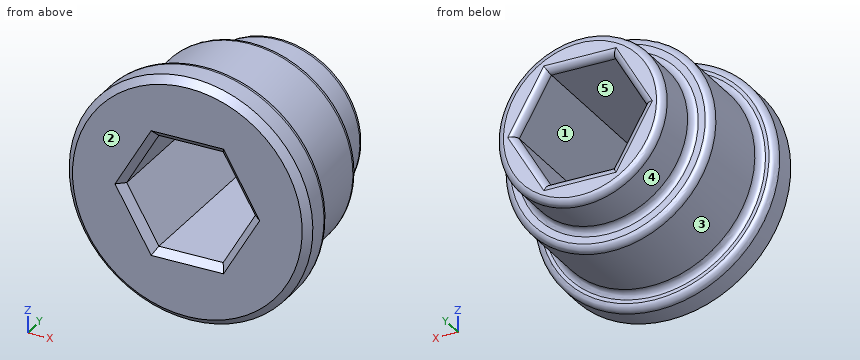
from build123d import *

# Parameters (mm, degrees)
SKETCH1_R           = 9.525
BOSS_EXTRUDE1_DEPTH = 7.9375
SKETCH2_R           = 7.62
BOSS_EXTRUDE2_DEPTH = 4.7625
SKETCH3_R           = 11.1125
BOSS_EXTRUDE3_DEPTH = 3.175
FILLET1_R           = 0.635
FILLET3_R           = 0.635
FILLET4_R           = 0.635
CHAMFER1_SIZE       = 0.635


with BuildPart() as part:
    # Sketch1 → Boss-Extrude1 (new body)
    with BuildSketch(Plane(origin=(0, 0, 0), x_dir=(1, 0, 0), z_dir=(0, 1, 0))):
        with Locations(Location((0, 0, 0), (0, 0, 270))):
            Circle(SKETCH1_R)
        Polygon((5.865878735, 0), (2.932939367, 5.08), (-2.932939367, 5.08), (-5.865878735, 0), (-2.932939367, -5.08), (2.932939367, -5.08), align=None, mode=Mode.SUBTRACT)
    extrude(amount=BOSS_EXTRUDE1_DEPTH)

    # Sketch2 → Boss-Extrude2 (add)
    with BuildSketch(Plane(origin=(0, 7.9375, 0), x_dir=(1, 0, 0), z_dir=(0, 1, 0))):
        with Locations(Location((0, 0, 0), (0, 0, 90))):
            Circle(SKETCH2_R)
        Polygon((-2.932939367, 5.08), (-5.865878735, 0), (-2.932939367, -5.08), (2.932939367, -5.08), (5.865878735, 0), (2.932939367, 5.08), align=None, mode=Mode.SUBTRACT)
    extrude(amount=BOSS_EXTRUDE2_DEPTH)

    # Sketch3 → Boss-Extrude3 (add)
    with BuildSketch(Plane.XZ):
        with Locations(Location((0, 0, 0), (0, 0, 270))):
            Circle(SKETCH3_R)
        Polygon((-2.932939367, 5.08), (2.932939367, 5.08), (5.865878735, 0), (2.932939367, -5.08), (-2.932939367, -5.08), (-5.865878735, 0), align=None, mode=Mode.SUBTRACT)
    extrude(amount=BOSS_EXTRUDE3_DEPTH)

    # Fillet1
    fillet1_edges = [part.edges().sort_by_distance(p)[0] for p in [
        (0, 0, -9.525),
        (0, 0, 11.1125),
    ]]
    fillet(fillet1_edges, radius=FILLET1_R)

    # Fillet3
    fillet3_edges = [part.edges().sort_by_distance(p)[0] for p in [
        (0, 12.7, -5.08),
        (-4.399409051, 12.7, -2.54),
        (-4.399409051, 12.7, 2.54),
        (0, 12.7, 5.08),
        (4.399409051, 12.7, 2.54),
        (4.399409051, 12.7, -2.54),
    ]]
    fillet(fillet3_edges, radius=FILLET3_R)

    # Fillet4
    fillet4_edges = [part.edges().sort_by_distance(p)[0] for p in [
        (0, 12.7, 7.62),
        (0, 7.9375, 7.62),
        (0, 7.9375, -9.525),
    ]]
    fillet(fillet4_edges, radius=FILLET4_R)

    # Chamfer1
    chamfer1_edges = [part.edges().sort_by_distance(p)[0] for p in [
        (0, -3.175, 11.1125),
        (-4.399409051, -3.175, 2.54),
        (-4.399409051, -3.175, -2.54),
        (0, -3.175, -5.08),
        (4.399409051, -3.175, -2.54),
        (4.399409051, -3.175, 2.54),
        (0, -3.175, 5.08),
    ]]
    chamfer(chamfer1_edges, length=CHAMFER1_SIZE)


solid = part.part
Geometry check sheet. Reference: the model listing, model coordinates, mm. Face numbers are marked on the shaded views. A direction names the side the tool comes from. Give positions to 0.01 mm unless a question says otherwise; leave off trailing zeros. Write each loop counter-clockwise with the first axis right and the second up, starting at its lowest first coordinate (ties: lowest second). Pieces come first, ordered by that corner, then holes. Notation, with made-up numbers: (-28.5, 46) - (-6.5, 46) arc R9 ccw to (-6.5, 58) - close; hole circle Ø8 at (61.25, 62). An arc over 180 degrees is marked (long way). Put each result on its own line as item: value.
1. Sectioned sample at A-A, the plane y = 6. Enter the section's corners in (x, z) (3 decimals), plus the area to 3 significant figures.
Ans:
outline: circle Ø19.05 at (0, 0); hole (-5.866, 0) - (-2.933, -5.08) - (2.933, -5.08) - (5.866, 0) - (2.933, 5.08) - (-2.933, 5.08) - close
area: 196 mm²
2. Go/stop test with flat-tipped pins: pin 1 (1.8 mm diameter, centred on x = 1, y = 4.5, fed in from +Z); pin 2 (1 mm diameter, centred on x = 7.5, y = 2.5, fed in from -Z); pin 3 (3 mm diameter, centred on x = 0.5, y = 4, fed in from -Z) (3 decimals). Record where each tip stops, or that it passes through.
Ans:
pin 1: stops at z = 9.52
pin 2: stops at z = -6.46
pin 3: stops at z = -9.525
3. Thickness scan on line 1 (Z direction, x = -0.25, y = 0.75); line 2 (Z direction, x = -3, y = 7); line 3 (Y direction, x = -4, z = 7.5) (1 decimal). Record the ranges inside material, lowest first.
Ans:
line 1: z = -9.52 to -5.08, 5.08 to 9.52
line 2: z = -9.04 to -4.96, 4.96 to 9.04
line 3: y = -3.2 to 7.9
4. Set-up check for the marked faces 4 and 5: record each of +Z, -Z, +X, -X, +Y, -Y from which the full face is reachable in a straight line by a thin tool's end or side.
Ans:
face 4: +Y
face 5: +Y, -Y
5. Draft check along X on the marked faces 1, 2 and 3. Enter one of: +X half, -X half, draft (parallel to the pull), parting line (faces both ways), or undercut.
Ans:
face 1: undercut
face 2: draft
face 3: parting line
